Input: part model. Units: mm. Frame: model coordinates. Face numbers are marked on the shaded views. Round coordinates to 2 decimals unless told otherwise and drop trailing zeros. Order: outer loops, then holes, each group sorted by start corner. A loop starts at its lowest first (then second) coordinate and runs counter-clockwise, first axis right, second up. Notation, with made-up numbers: (24.25, 76.5) -> (51.25, 76.5) arc R24 ccw to (51.25, 86.5) -> close; hole circle Ø10 at (5.5, 60). An arc over 180 degrees is marked (long way). Answer as CSV lines item,"result". Start each with the question number.
1) Section query A-A, the plane x = 49. Output: boundary loops of the cut face in (y, z).
2) Section query B-B, the plane y = 71. Output: boundary loops of the cut face in (x, z).
3) Line query: L1, parallel to X at y = 10, z = 2; L2, parallel to X at y = 12.5, z = 4.7; L3, parallel to Y at x = 49, z = 3.45. Output: solid intervals per line, ascending.
4) Section query D-D, the plane z = 1.05. Output: boundary loops of the cut face in (x, y), and give its area (3 significant figures).
5) Section query C-C, the plane z = 4.95. Output: boundary loops of the cut face in (x, y), and give its area (3 significant figures).
6) Mould query, pull axis Z, two halves, no side actions, for the marked faces 1, 2 and 3. Classes: +Z half, -Z half, draft (parallel to the pull), parting line (faces both ways), or undercut.
7) First-contact query: P1, Ø3, axis at x = 9, y = 32, coming from the -Z side; P2, Ø10.5, axis at x = 49, y = 10, coming from the +Z side. Flat tips, straight axial feed; report the tip coordinate or a pass-through.
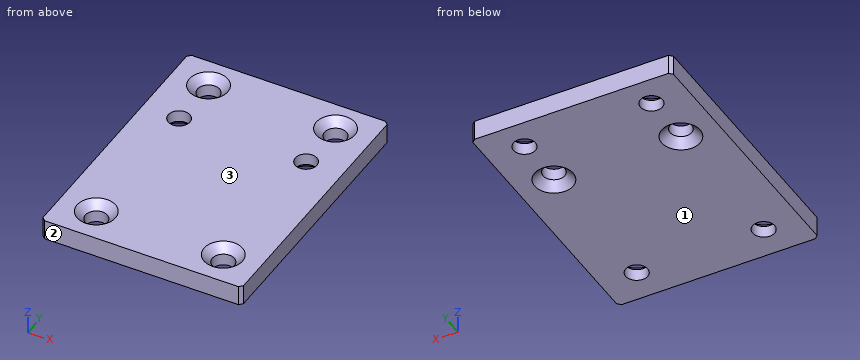
Autodesk Inventor part; units mm, degrees
ref_plane "YZ Plane" through (0, 0, 0) normal (1, 0, 0) x (0, 1, 0)
ref_plane "XZ Plane" through (0, 0, 0) normal (0, 1, 0) x (-1, 0, 0)
ref_plane "XY Plane" through (0, 0, 0) normal (0, 0, 1) x (1, 0, 0)
sketch "Sketch1" plane through (0, 0, 0) normal (0, 0, 1) x (1, 0, 0)
  line L0 (0, 0) -> (60, 0)
  line L1 (60, 0) -> (60, 80)
  line L2 (60, 80) -> (0, 80)
  line L3 (0, 80) -> (0, 0)
  dimension "d0" = 80
  dimension "d1" = 60
extrude "Extrusion1" add sketch "Sketch1" along normal blind 6
sketch "Sketch2" plane through (0, 0, 6) normal (0, 0, 1) x (1, 0, 0)
  line L0 (0, 0) -> (0, 80)
  line L1 (60, 0) -> (0, 0)
  point P0 (11, 71)
  point P1 (49, 71)
  point P2 (11, 10)
  point P3 (49, 10)
  dimension "d4" = 11
  dimension "d5" = 49
  dimension "d6" = 10
  dimension "d7" = 11
  dimension "d8" = 49
  dimension "d13" = 71
  dimension "d14" = 71
  dimension "d15" = 10
hole "Hole1" at (11, 71, 6) at (49, 71, 6) at (11, 10, 6) at (49, 10, 6) direction (0, 0, -1) diameter 6.6 depth 6 tip angle 118 countersink diameter 11.5 countersink angle 90
sketch "Sketch3" plane through (0, 0, 0) normal (0, 0, -1) x (-1, 0, 0)
  line L0 (0, 0) -> (-60, 0)
  line L1 (-60, 0) -> (-60, 80)
  point P0 (-49, 55)
  point P1 (-11, 55)
  dimension "d26" = 55
  dimension "d27" = 55
  dimension "d28" = 11
  dimension "d29" = 49
hole "Hole2" at (49, 55, 0) at (11, 55, 0) direction (0, 0, 1) diameter 6.5 depth 6 tip angle 118 countersink diameter 11.5 countersink angle 90
chamfer "Chamfer2" distance 1 angle 45 4 edges at (60, 0, 3) (60, 80, 3) (0, 80, 3) (0, 0, 3)
properties part number "TRASEIRA DA CABINE" material "Carbon Steel"
Findings:
1,outline,"(0, 0) -> (6.7, 0) -> (6.7, 3.55) -> (4.25, 6) -> (0, 6) -> close; (13.3, 0) -> (49.25, 0) -> (51.75, 2.5) -> (51.75, 6) -> (15.75, 6) -> (13.3, 3.55) -> close; (58.25, 2.5) -> (60.75, 0) -> (67.7, 0) -> (67.7, 3.55) -> (65.25, 6) -> (58.25, 6) -> close; (74.3, 0) -> (80, 0) -> (80, 6) -> (76.75, 6) -> (74.3, 3.55) -> close"
2,outline,"(0, 0) -> (7.7, 0) -> (7.7, 3.55) -> (5.25, 6) -> (0, 6) -> close; (14.3, 0) -> (45.7, 0) -> (45.7, 3.55) -> (43.25, 6) -> (16.75, 6) -> (14.3, 3.55) -> close; (52.3, 0) -> (60, 0) -> (60, 6) -> (54.75, 6) -> (52.3, 3.55) -> close"
3,L1,"x = 0 to 7.7, 14.3 to 45.7, 52.3 to 60"
3,L2,"x = 0 to 7.32, 14.68 to 45.32, 52.68 to 60"
3,L3,"y = 0 to 6.7, 13.3 to 51.75, 58.25 to 67.7, 74.3 to 80"
4,outline,"(0, 1) -> (1, 0) -> (59, 0) -> (60, 1) -> (60, 79) -> (59, 80) -> (1, 80) -> (0, 79) -> close; hole circle Ø9.4 at (11, 55); hole circle Ø6.6 at (11, 10); hole circle Ø6.6 at (11, 71); hole circle Ø9.4 at (49, 55); hole circle Ø6.6 at (49, 10); hole circle Ø6.6 at (49, 71)"
4,area,"4,520 mm^2"
5,outline,"(0, 1) -> (1, 0) -> (59, 0) -> (60, 1) -> (60, 79) -> (59, 80) -> (1, 80) -> (0, 79) -> close; hole circle Ø9.4 at (11, 10); hole circle Ø9.4 at (11, 71); hole circle Ø6.5 at (11, 55); hole circle Ø9.4 at (49, 10); hole circle Ø9.4 at (49, 71); hole circle Ø6.5 at (49, 55)"
5,area,"4,450 mm^2"
6,face 1,"-Z half"
6,face 2,"draft"
6,face 3,"+Z half"
7,P1,"stops at z = 0"
7,P2,"stops at z = 5.5"
